```python
from build123d import *

# Parameters (mm, degrees)
SKETCH_1_R      = 4
SKETCH_1_R_2    = 2
EXTRUDE_1_DEPTH = 3


with BuildPart() as part:
    # 草图1 → 凸台-拉伸1 (new body)
    with BuildSketch(Plane.XY):
        Polygon((27.370057685, 11), (27.370057685, 12.5), (24.770057685, 12.5), (24.770057685, 11), (21.770057685, 11), (21.770057685, 8), (24.770057685, 8), (24.770057685, 6.5), (27.370057685, 6.5), (27.370057685, 8), (29.870057685, 8), (29.870057685, 4), (32.870057685, 4), (32.870057685, 0), (32.870057685, -4), (29.870057685, -4), (29.870057685, -8), (27.370057685, -8), (27.370057685, -6.5), (24.770057685, -6.5), (24.770057685, -8), (21.770057685, -8), (21.770057685, -11), (24.770057685, -11), (24.770057685, -12.5), (27.370057685, -12.5), (27.370057685, -11), (29.870057685, -11), (29.870057685, -22), (-26.129942315, -22), (-26.129942315, 22), (29.870057685, 22), (29.870057685, 11), align=None)
        Circle(SKETCH_1_R, mode=Mode.SUBTRACT)
        with Locations((0, -19)):
            Circle(SKETCH_1_R_2, mode=Mode.SUBTRACT)
        with Locations((-13.435028843, -13.435028843)):
            Circle(SKETCH_1_R_2, mode=Mode.SUBTRACT)
        with Locations((-19, 0)):
            Circle(SKETCH_1_R_2, mode=Mode.SUBTRACT)
        with Locations((-13.435028843, 13.435028843)):
            Circle(SKETCH_1_R_2, mode=Mode.SUBTRACT)
        with Locations((0, 19)):
            Circle(SKETCH_1_R_2, mode=Mode.SUBTRACT)
        with Locations((13.435028843, 13.435028843)):
            Circle(SKETCH_1_R_2, mode=Mode.SUBTRACT)
        with Locations((19, 0)):
            Circle(SKETCH_1_R_2, mode=Mode.SUBTRACT)
        with Locations((13.435028843, -13.435028843)):
            Circle(SKETCH_1_R_2, mode=Mode.SUBTRACT)
    extrude(amount=EXTRUDE_1_DEPTH)


solid = part.part
```
Geometry: final body of the model. Coordinates: model frame, mm. A direction names the side the tool comes from. Round coordinates to 2 decimals unless told otherwise and drop trailing zeros. Write each loop counter-clockwise with the first axis right and the second up, starting at its lowest first coordinate (ties: lowest second). Pieces come first, ordered by that corner, then holes. Notation, with made-up numbers: (88, -21) -> (136, -21) arc R18 ccw to (136, 8) -> close; hole circle Ø1 at (22.25, -27.5). An arc over 180 degrees is marked (long way). Return JSON: item names as keys, results as strings.
Q1. Ray query, line 1 (Y direction, x = 0, z = 2.45); line 2 (Y direction, x = 25.5, z = 0.25); line 3 (Y direction, x = -19, z = 1.05). Return the intervals inside material, ascending.
From the geometry:
{"line 1": "-22 to -21, -17 to -4, 4 to 17, 21 to 22", "line 2": "-22 to -12.5, -6.5 to 6.5, 12.5 to 22", "line 3": "-22 to -2, 2 to 22"}
Q2. Section D-D on x = 19. Return the cut outline in (y, z).
From the geometry:
{"outline": "(-22, 0) -> (-2, 0) -> (-2, 3) -> (-22, 3) -> close; (2, 0) -> (22, 0) -> (22, 3) -> (2, 3) -> close"}
Q3. First-contact query: pin 1 Ø0.9 at (y, z) = (10, 1.5) entering from +X. Flat tip, straight axial feed; report the tip coordinate or a pass-through.
From the geometry:
{"pin 1": "x = 21.77"}
Q4. Section A-A on y = -19. Return the cut outline in (x, z).
From the geometry:
{"outline": "(-26.13, 0) -> (-2, 0) -> (-2, 3) -> (-26.13, 3) -> close; (2, 0) -> (29.87, 0) -> (29.87, 3) -> (2, 3) -> close"}
Q5. Set-up query: faces 1 (the flat face through (21.77, -9, 1)), 2 (the flat face through (31, -4, 1)), 3 (the flat face through (27.37, -7, 1)), 4 (the flat face through (29.87, 6, 1)). Return all of +Z, -Z, +X, -X, +Y, -Y with unobstructed straight access to the full face (end or side cutting, diameter ignored); none if empty.
From the geometry:
{"face 1": "+Z, -Z, +X", "face 2": "+Z, -Z, +X, -Y", "face 3": "+Z, -Z", "face 4": "+Z, -Z, +X, +Y"}
Q6. Mould query, pull axis X, two halves, no side actions, for faces 5 (the cylindrical face through (17.4, -1.2, 1.5)), 6 (the flat face through (31, 4, 1)), 7 (the flat face through (-26.13, 0, 1)). Classes: +X half, -X half, draft (parallel to the pull), parting line (faces both ways), or undercut.
From the geometry:
{"face 5": "undercut", "face 6": "draft", "face 7": "-X half"}
Q7. Section B-B on y = 0. Return the cut outline in (x, z).
From the geometry:
{"outline": "(-26.13, 0) -> (-21, 0) -> (-21, 3) -> (-26.13, 3) -> close; (-17, 0) -> (-4, 0) -> (-4, 3) -> (-17, 3) -> close; (4, 0) -> (17, 0) -> (17, 3) -> (4, 3) -> close; (21, 0) -> (32.87, 0) -> (32.87, 3) -> (21, 3) -> close"}
Q8. Section C-C on x = 0. Return the cut outline in (y, z), and give its area (3 significant figures).
From the geometry:
{"outline": "(-22, 0) -> (-21, 0) -> (-21, 3) -> (-22, 3) -> close; (-17, 0) -> (-4, 0) -> (-4, 3) -> (-17, 3) -> close; (4, 0) -> (17, 0) -> (17, 3) -> (4, 3) -> close; (21, 0) -> (22, 0) -> (22, 3) -> (21, 3) -> close", "area": "84.0 mm2"}
